Check sheet for the modelled part. Datum: model origin and axes. Units: mm. A direction names the side the tool comes from. Round coordinates to 2 decimals unless told otherwise and drop trailing zeros. Loops run counter-clockwise (first coordinate to the right, second up) from the corner with the lowest first, then second, coordinate; pieces in that order, holes last. Notation, with made-up numbers: (68, -22) -> (88, -22) arc R19 cw to (88, 5) -> close; hole circle Ø2 at (37.25, 56). An arc over 180 degrees is marked (long way). One line per item, written item: value. Start each with the question number.
1. Cross-section at C-C on z = 6.5. Record the cut outline in (x, y), then the cut area to 3 significant figures.
2. Cross-section at A-A on y = 21.5. Record the cut outline in (x, z), then the cut area to 3 significant figures.
3. Release check for a two-part mould opening along Z. For faces 4 (the face through (20.111, 47.535, -9.086)), 5 (the face through (12.5, 14, -12)), 6 (the face through (22, 25, 12.5)) record: +Z half, -Z half, draft (parallel to the pull), parting line (faces both ways), or undercut.
4. Go/stop test with flat-tipped pins: pin 1 (2.5 mm diameter, centred on y = 25, z = -21, fed in from +X); pin 2 (2 mm diameter, centred on x = -2.5, y = 34.5, fed in from -Z); pin 3 (1.5 mm diameter, centred on x = -23.5, z = 10, fed in from -Y). Record where each tip stops, or that it passes through.
5. Set-up check for faces 1 (the face through (7, 25, -21)), 2 (the face through (22, 35, 7.5)), 3 (the face through (21, 23, -6.5)): record each of +Z, -Z, +X, -X, +Y, -Y from which the full face is reachable in a straight line by a thin tool's end or side.
6. Cross-section at B-B on x = 0. Record the cut outline in (y, z), then the cut area to 3 significant figures.
7. Material ranges on L1, parallel to Y at x = 22.5, z = -3; L2, parallel to X at y = 4, z = -13.5; L3, parallel to X at y = 4.5, z = 4.5, recorded low to high.
8. Cross-section at D-D on y = 42.5. Record the cut outline in (x, z).
from build123d import *

# Parameters (mm, degrees)
SKETCH2_R            = 27.5
BOSS_EXTRUDE1_DEPTH  = 50
SKETCH3_R            = 26
CUT_EXTRUDE1_DEPTH   = 51
SKETCH7_R            = 18.25
BOSS_EXTRUDE3_DEPTH  = 50
SKETCH8_R            = 16.75
CUT_EXTRUDE3_DEPTH   = 51
SKETCH9_W            = 59.961193285
SKETCH9_H            = 28.516087398
CUT_EXTRUDE4_DEPTH   = 51
SKETCH10_W           = 1.5
SKETCH10_H           = 12.5
BOSS_EXTRUDE4_DEPTH  = 50
BOSS_EXTRUDE5_DEPTH  = 5
BOSS_EXTRUDE6_DEPTH  = 6.5
SKETCH12_W           = 14
SKETCH12_H           = 20
SKETCH12_W_2         = 20
SKETCH12_H_2         = 14
CUT_EXTRUDE6_DEPTH   = 15
SKETCH14_W           = 14
SKETCH14_H           = 20
CUT_EXTRUDE7_DEPTH   = 45
SKETCH15_W           = 16.605878589
SKETCH15_H           = 22.2356131
CUT_EXTRUDE8_DEPTH   = 15
BOSS_EXTRUDE8_DEPTH  = 4.5
BOSS_EXTRUDE9_DEPTH  = 2
BOSS_EXTRUDE10_DEPTH = 2
BOSS_EXTRUDE15_DEPTH = 24
BOSS_EXTRUDE17_DEPTH = 10
SKETCH26_W           = 5
SKETCH26_H           = 18
BOSS_EXTRUDE18_DEPTH = 10
SKETCH27_W           = 7.75
SKETCH27_H           = 14
BOSS_EXTRUDE19_DEPTH = 5
SKETCH29_W           = 14
SKETCH29_H           = 20
CUT_EXTRUDE9_DEPTH   = 8
SKETCH30_W           = 2
SKETCH30_H           = 20
BOSS_EXTRUDE20_DEPTH = 10


with BuildPart() as part:
    # Sketch2 → Boss-Extrude1 (new body)
    with BuildSketch(Plane(origin=(0, 0, 0), x_dir=(1, 0, 0), z_dir=(0, 1, 0))):
        Circle(SKETCH2_R)
    extrude(amount=BOSS_EXTRUDE1_DEPTH)

    # Sketch3 → Cut-Extrude1 (cut, through all)
    with BuildSketch(Plane(origin=(0, 50, 0), x_dir=(1, 0, 0), z_dir=(0, 1, 0))):
        Circle(SKETCH3_R)
    extrude(amount=-CUT_EXTRUDE1_DEPTH, mode=Mode.SUBTRACT)


with BuildPart() as body_2:
    # Sketch7 → Boss-Extrude3 (new body)
    with BuildSketch(Plane(origin=(0, 50, 0), x_dir=(1, 0, 0), z_dir=(0, 1, 0))):
        Circle(SKETCH7_R)
    extrude(amount=-BOSS_EXTRUDE3_DEPTH)

    # Sketch8 → Cut-Extrude3 (cut, through all)
    with BuildSketch(Plane(origin=(0, 50, 0), x_dir=(1, 0, 0), z_dir=(0, 1, 0))):
        Circle(SKETCH8_R)
    extrude(amount=-CUT_EXTRUDE3_DEPTH, mode=Mode.SUBTRACT)


with BuildPart() as cut_extrude4_tool:
    # Sketch9 → Cut-Extrude4 (new body, through all)
    with BuildSketch(Plane(origin=(0, 50, 0), x_dir=(1, 0, 0), z_dir=(0, 1, 0))):
        with Locations((-0.477134602, -14.258043699)):
            Rectangle(SKETCH9_W, SKETCH9_H)
    extrude(amount=-CUT_EXTRUDE4_DEPTH)


with BuildPart() as part_1:
    add(part.part)

    # Cut-Extrude4: cut by cut_extrude4_tool
    add(cut_extrude4_tool.part, mode=Mode.SUBTRACT)



with BuildPart() as body_2_1:
    add(body_2.part)

    # Cut-Extrude4: cut by cut_extrude4_tool
    add(cut_extrude4_tool.part, mode=Mode.SUBTRACT)


with BuildPart() as part_2:
    add(part_1.part)

    add(body_2_1.part)  # Boss-Extrude4 merges body 2
    # Sketch10 → Boss-Extrude4 (add)
    with BuildSketch(Plane(origin=(0, 50, 0), x_dir=(1, 0, 0), z_dir=(0, 1, 0))):
        with Locations((-26.75, -6.25)):
            Rectangle(SKETCH10_W, SKETCH10_H)
        with Locations((-17.5, -6.25)):
            Rectangle(SKETCH10_W, SKETCH10_H)
        with Locations((17.5, -6.25)):
            Rectangle(SKETCH10_W, SKETCH10_H)
        with Locations((26.75, -6.25)):
            Rectangle(SKETCH10_W, SKETCH10_H)
    extrude(amount=-BOSS_EXTRUDE4_DEPTH)

    # Sketch11 → Boss-Extrude5 (add)
    with BuildSketch(Plane(origin=(0, 50, 0), x_dir=(1, 0, 0), z_dir=(0, 1, 0))):
        with BuildLine():
            Line((16.760723177, 7.220848882), (23.556882961, 11.003329731))
            ThreePointArc((23.556882961, 11.003329731), (25.38187303, 5.63564739), (26, 0))
            Line((26, 0), (26, -12.5))
            Line((26, -12.5), (18.25, -12.5))
            Line((18.25, -12.5), (18.25, 0))
            ThreePointArc((18.25, 0), (17.873803428, 3.686414384), (16.760723177, 7.220848882))
        make_face()
    extrude(amount=-BOSS_EXTRUDE5_DEPTH)

    # Sketch13 → Boss-Extrude6 (add)
    with BuildSketch(Plane.XZ):
        with BuildLine():
            Line((18.25, 0), (18.25, 12.5))
            Line((18.25, 12.5), (26, 12.5))
            Line((26, 12.5), (26, 0))
            ThreePointArc((26, 0), (25.38187303, -5.63564739), (23.556882961, -11.003329731))
            Line((23.556882961, -11.003329731), (16.760723177, -7.220848882))
            ThreePointArc((16.760723177, -7.220848882), (17.873803428, -3.686414384), (18.25, 0))
        make_face()
    extrude(amount=-BOSS_EXTRUDE6_DEPTH)

    # Sketch12 → Cut-Extrude6 (cut)
    with BuildSketch(Plane(origin=(27.5, 0, 0), x_dir=(0, 0, -1), z_dir=(1, 0, 0))):
        with Locations((-0.5, 35)):
            Rectangle(SKETCH12_W, SKETCH12_H)
        with Locations((2.5, 13.5)):
            Rectangle(SKETCH12_W_2, SKETCH12_H_2)
    extrude(amount=-CUT_EXTRUDE6_DEPTH, mode=Mode.SUBTRACT)

    # Sketch14 → Cut-Extrude7 (cut)
    with BuildSketch(Plane.XY.offset(12.5)):
        with Locations((0, 25)):
            Rectangle(SKETCH14_W, SKETCH14_H)
    extrude(amount=-CUT_EXTRUDE7_DEPTH, mode=Mode.SUBTRACT)

    # Sketch15 → Cut-Extrude8 (cut)
    with BuildSketch(Plane.ZY.offset(27.5)):
        with Locations((15.802939295, 43.11780655)):
            Rectangle(SKETCH15_W, SKETCH15_H)
    extrude(amount=-CUT_EXTRUDE8_DEPTH, mode=Mode.SUBTRACT)

    # Sketch17 → Boss-Extrude8 (add)
    with BuildSketch(Plane(origin=(0, 25, 0), x_dir=(1, 0, 0), z_dir=(0, 1, 0))):
        with BuildLine():
            Line((26.720778432, 6.5), (17.053225501, 6.5))
            ThreePointArc((17.053225501, 6.5), (17.948312809, 3.304628164), (18.25, 0))
            Line((18.25, 0), (18.25, -7.5))
            Line((18.25, -7.5), (27.5, -7.5))
            Line((27.5, -7.5), (27.5, 0))
            ThreePointArc((27.5, 0), (27.304499692, 3.273270011), (26.720778432, 6.5))
        make_face()
    extrude(amount=-BOSS_EXTRUDE8_DEPTH)

    # Sketch18 → Boss-Extrude9 (add)
    with BuildSketch(Plane.XZ.offset(-35)):
        with BuildLine():
            Line((-7, -16.854153791), (-7, -25.039968051))
            ThreePointArc((-7, -25.039968051), (0, -26), (7, -25.039968051))
            Line((7, -25.039968051), (7, -16.854153791))
            ThreePointArc((7, -16.854153791), (0, -18.25), (-7, -16.854153791))
        make_face()
    extrude(amount=-BOSS_EXTRUDE9_DEPTH)

    # Sketch19 → Boss-Extrude10 (add)
    with BuildSketch(Plane(origin=(0, 15, 0), x_dir=(1, 0, 0), z_dir=(0, 1, 0))):
        with BuildLine():
            Line((7, 25.039968051), (7, 16.854153791))
            ThreePointArc((7, 16.854153791), (0, 18.25), (-7, 16.854153791))
            Line((-7, 16.854153791), (-7, 25.039968051))
            ThreePointArc((-7, 25.039968051), (0, 26), (7, 25.039968051))
        make_face()
    extrude(amount=-BOSS_EXTRUDE10_DEPTH)

    # Sketch24 → Boss-Extrude15 (add)
    with BuildSketch(Plane(origin=(0, 37, 0), x_dir=(1, 0, 0), z_dir=(0, 1, 0))):
        with BuildLine():
            Line((8.237316258, 24.660628963), (8.237316258, 16.285242426))
            ThreePointArc((8.237316258, 16.285242426), (7.6239666, 16.581243418), (7, 16.854153791))
            Line((7, 16.854153791), (7, 25.039968051))
            ThreePointArc((7, 25.039968051), (7.621018713, 24.857998185), (8.237316258, 24.660628963))
        make_face()
    extrude(amount=-BOSS_EXTRUDE15_DEPTH)

    # Sketch25 → Boss-Extrude17 (add)
    with BuildSketch(Plane(origin=(27.5, 0, 0), x_dir=(0, 0, -1), z_dir=(1, 0, 0))):
        Polygon((-7.5, 45), (-12.5, 45), (-12.5, 25), (-12.5, 20.5), (-7.5, 20.5), (-7.5, 25), align=None)
    extrude(amount=-BOSS_EXTRUDE17_DEPTH)

    # Sketch26 → Boss-Extrude18 (add)
    with BuildSketch(Plane.ZY.offset(27.5)):
        with Locations((10, 23)):
            Rectangle(SKETCH26_W, SKETCH26_H)
    extrude(amount=-BOSS_EXTRUDE18_DEPTH)

    # Sketch27 → Boss-Extrude19 (add)
    with BuildSketch(Plane.XY.offset(12.5)):
        with Locations((22.125, 13.5)):
            Rectangle(SKETCH27_W, SKETCH27_H)
    extrude(amount=-BOSS_EXTRUDE19_DEPTH)

    # Sketch29 → Cut-Extrude9 (cut)
    with BuildSketch(Plane.ZY.offset(27.5)):
        with Locations((-4.5, 20)):
            Rectangle(SKETCH29_W, SKETCH29_H)
    extrude(amount=-CUT_EXTRUDE9_DEPTH, mode=Mode.SUBTRACT)

    # Sketch30 → Boss-Extrude20 (add)
    with BuildSketch(Plane.ZY.offset(27.5)):
        with Locations((3.5, 20)):
            Rectangle(SKETCH30_W, SKETCH30_H)
    extrude(amount=-BOSS_EXTRUDE20_DEPTH)


solid = part_2.part
Taken from the geometry:
1. outline: (-27.5, 0) -> (-26, 0) -> (-26, 50) -> (-27.5, 50) -> close; (-18.25, 0) -> (-16.75, 0) -> (-16.75, 50) -> (-18.25, 50) -> close; (16.75, 0) -> (27.5, 0) -> (27.5, 6.5) -> (16.75, 6.5) -> close; (16.75, 20.5) -> (27.5, 20.5) -> (27.5, 25) -> (16.75, 25) -> close; (16.75, 45) -> (27.5, 45) -> (27.5, 50) -> (16.75, 50) -> close
1. area: 322 mm2
2. outline: (-27.5, 2.5) -> (-18.25, 2.5) -> (-18.25, 0) arc R18.25 ccw to (-7, -16.85) -> (-7, -15.22) arc R16.75 cw to (-16.75, 0) -> (-16.75, 12.5) -> (-27.5, 12.5) -> close; (-24.98, -11.5) arc R27.5 ccw to (-7, -26.59) -> (-7, -25.04) arc R26 cw to (-23.32, -11.5) -> close; (7, -26.59) arc R27.5 ccw to (27.5, 0) -> (27.5, 12.5) -> (16.75, 12.5) -> (16.75, 0) arc R16.75 cw to (7, -15.22) -> close; hole (-26, 4.5) -> (-18.25, 4.5) -> (-18.25, 7.5) -> (-26, 7.5) -> close; hole (8.24, -24.66) arc R26 ccw to (25.17, -6.5) -> (17.05, -6.5) arc R18.25 cw to (8.24, -16.29) -> close
2. area: 432 mm2
3. face 4: undercut
3. face 5: draft
3. face 6: +Z half
4. pin 1: stops at x = 19.14
4. pin 2: stops at z = -27.45
4. pin 3: stops at y = 14
5. face 1: +Z, -Z
5. face 2: +X
5. face 3: none
6. outline: (0, -27.5) -> (15, -27.5) -> (15, -16.75) -> (0, -16.75) -> (0, -18.25) -> (13, -18.25) -> (13, -26) -> (0, -26) -> close; (35, -27.5) -> (50, -27.5) -> (50, -26) -> (37, -26) -> (37, -18.25) -> (50, -18.25) -> (50, -16.75) -> (35, -16.75) -> close
6. area: 121 mm2
7. L1: y = 0 to 6.5, 20.5 to 25, 45 to 50
7. L2: x = -23.96 to -22.22, -12.28 to -9.92, 9.92 to 12.28, 22.22 to 23.96
7. L3: x = -27.5 to -26, -18.25 to -16.75, 16.75 to 27.5
8. outline: (-27.5, 0) arc R27.5 ccw to (26.72, -6.5) -> (25.17, -6.5) arc R26 cw to (-26, 0) -> (-26, 7.5) -> (-27.5, 7.5) -> close; (-18.25, 0) arc R18.25 ccw to (17.05, -6.5) -> (15.44, -6.5) arc R16.75 cw to (-16.75, 0) -> (-16.75, 7.5) -> (-18.25, 7.5) -> close; (16.75, 7.5) -> (27.5, 7.5) -> (27.5, 12.5) -> (16.75, 12.5) -> close
